Drawing for the job (mm, zero at the part's lowest x, y, z). Round coordinates to 2 decimals unless told otherwise and drop trailing zeros. Loops run counter-clockwise (first coordinate to the right, second up) from the corner with the lowest first, then second, coordinate; pieces in that order, holes last. Notation, with made-up numbers: M -30.5,85.25 L 13.5,85.25 A11 ccw 13.5,89.25 Z; hole C 54.5,25 d11. An arc over 180 degrees is marked long. Answer in a Markdown table with one row per item.
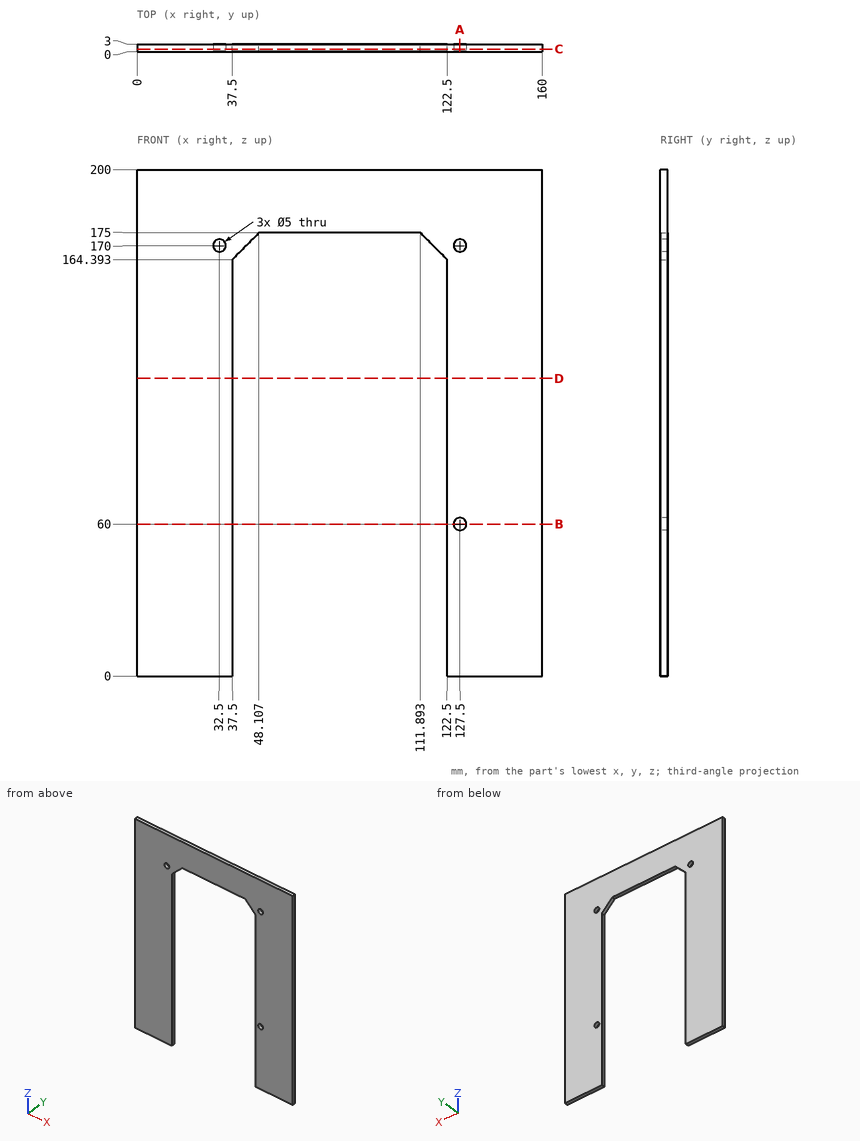
1. Saw through at B-B (z = 60). Write the cut outline in (x, y), and give its area (3 significant figures).
Verdict:
| item | result |
|---|---|
| outline | M 0,0 L 37.5,0 L 37.5,3 L 0,3 Z; M 122.5,0 L 125,0 L 125,3 L 122.5,3 Z; M 130,0 L 160,0 L 160,3 L 130,3 Z |
| area | 210 mm² |
2. Saw through at C-C (y = 1). Write the cut outline in (x, z).
Verdict:
| item | result |
|---|---|
| outline | M 0,0 L 37.5,0 L 37.5,164.39 L 48.11,175 L 111.89,175 L 122.5,164.39 L 122.5,0 L 160,0 L 160,200 L 0,200 Z; hole C 32.5,170 d5; hole C 127.5,60 d5; hole C 127.5,170 d5 |
3. Saw through at D-D (z = 117.5). Write the cut outline in (x, y).
Verdict:
| item | result |
|---|---|
| outline | M 0,0 L 37.5,0 L 37.5,3 L 0,3 Z; M 122.5,0 L 160,0 L 160,3 L 122.5,3 Z |
4. Pin check, flat tips, straight feed: pin 1 (3 mm diameter, centred on x = 127.5, z = 170, fed in from +Y); pin 2 (1.5 mm diameter, centred on y = 2, z = 46, fed in from -X); pin 3 (1.5 mm diameter, centred on x = 88, y = 1.5, fed in from -Z). Stop position of each tip, or through.
Verdict:
| item | result |
|---|---|
| pin 1 | passes through |
| pin 2 | stops at x = 0 |
| pin 3 | stops at z = 175 |
5. Saw through at A-A (x = 127.5). Write the cut outline in (y, z).
Verdict:
| item | result |
|---|---|
| outline | M 0,0 L 3,0 L 3,57.5 L 0,57.5 Z; M 0,62.5 L 3,62.5 L 3,167.5 L 0,167.5 Z; M 0,172.5 L 3,172.5 L 3,200 L 0,200 Z |
6. Wall check: probe 1 along X at (y, z) = (0.95, 60); probe 2 along Z at (x, y) = (127.5, 1.05); probe 3 along X at (y, z) = (1.65, 10). Give the ranges that are in metal, low to high.
Verdict:
| item | result |
|---|---|
| probe 1 | x = 0 to 37.5, 122.5 to 125, 130 to 160 |
| probe 2 | z = 0 to 57.5, 62.5 to 167.5, 172.5 to 200 |
| probe 3 | x = 0 to 37.5, 122.5 to 160 |
